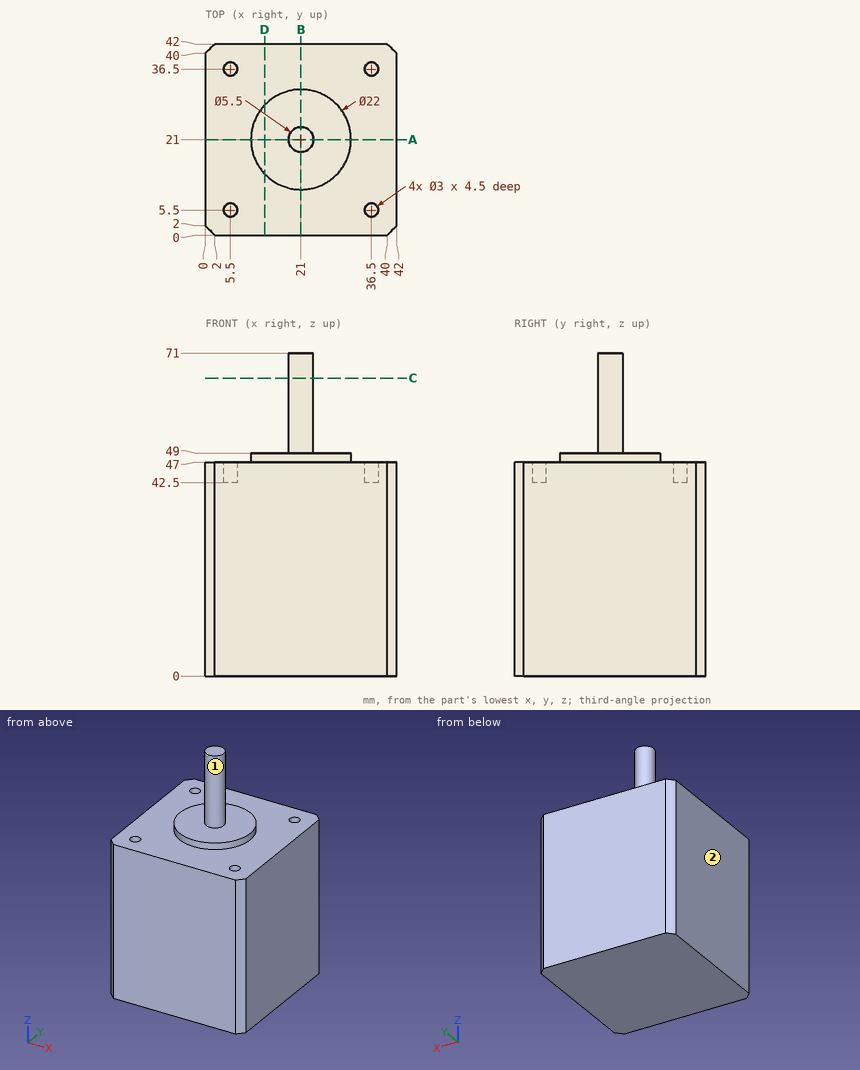
The drawing under review shows one solid part. Ordinate dimensions are in mm from its lowest x, y, z. A direction names the side the tool comes from. Round coordinates to 2 decimals unless told otherwise and drop trailing zeros. Write each loop counter-clockwise with the first axis right and the second up, starting at its lowest first coordinate (ties: lowest second). Pieces come first, ordered by that corner, then holes.
(1) Insertion check: pin 1 (4 mm diameter, centred on x = 5.5, y = 5.5, fed in from +Z); pin 2 (2 mm diameter, centred on x = 21.5, y = 26.5, fed in from -Z); pin 3 (2.5 mm diameter, centred on x = 36.5, y = 36.5, fed in from +Z); pin 4 (4 mm diameter, centred on x = 32, y = 16.5, fed in from +Z). Each pin has a flat end and moves straight along its axis. Give the tip position at first contact, or say it passes through.
(2) Machinability: for the marked faces 1 and 2, which of the approach directions +Z, -Z, +X, -X, +Y, -Y give a long, thin tool a straight path to every point of the face, cutting with its end or side? Answer none if there is none.
(3) We need section D-D on x = 13. Give the boundary of the cut face in (y, z).
(4) Wall thickness on L1, parallel to X at y = 5.5, z = 43.75; L2, parallel to Y at x = 5, z = 44: over which ranges is each line inside the solid? List them lowest first.
(5) We need section A-A on y = 21. Give the boundary of the cut face in (x, z), and give its area (3 significant figures).
(6) We need section C-C on z = 65.5. Give the boundary of the cut face in (x, y).
Findings below:
1. pin 1: stops at z = 47
1. pin 2: stops at z = 0
1. pin 3: stops at z = 42.5
1. pin 4: stops at z = 49
2. face 1: +Z
2. face 2: +Z, -Z, -X, +Y, -Y
3. outline: (0, 0) - (42, 0) - (42, 47) - (28.55, 47) - (28.55, 49) - (13.45, 49) - (13.45, 47) - (0, 47) - close
4. L1: x = 0 to 4, 7 to 35, 38 to 42
4. L2: y = 0 to 4.09, 6.91 to 35.09, 37.91 to 42
5. outline: (0, 0) - (42, 0) - (42, 47) - (32, 47) - (32, 49) - (23.75, 49) - (23.75, 71) - (18.25, 71) - (18.25, 49) - (10, 49) - (10, 47) - (0, 47) - close
5. area: 2,140 mm2
6. outline: circle Ø5.5 at (21, 21)
